The figure shows three views and two pictorial views of one solid part (mm, origin at its lowest corner). Answer the questions. Round coordinates to 2 decimals unless told otherwise and drop trailing zeros. Order: outer loops, then holes, each group sorted by start corner. A loop starts at its lowest first (then second) coordinate and runs counter-clockwise, first axis right, second up. Notation, with made-up numbers: (-23.75, 30.25) - (-5.75, 30.25) arc R31 cw to (-5.75, 60.25) - close; hole circle Ø5 at (81, 57). An arc over 180 degrees is marked (long way). Write item = value, one per line.
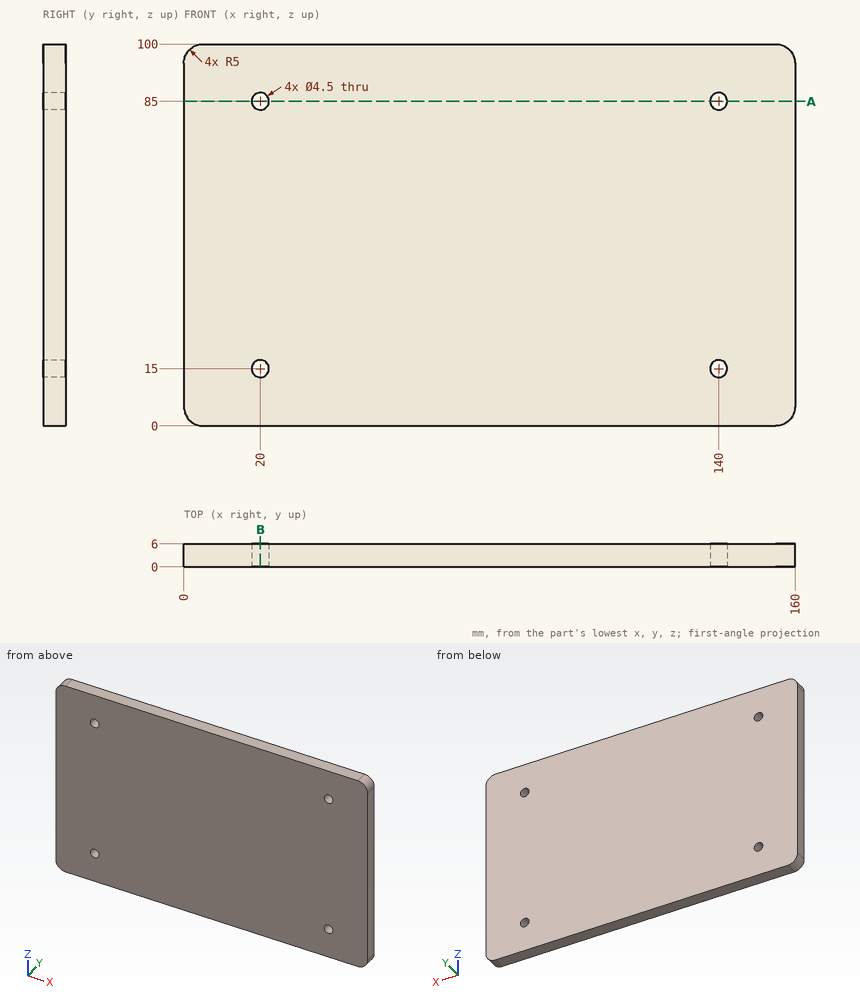
Q1. Section A-A on z = 85 is taken. Determine the outline of the cut face in (x, y).
Model answer:
outline = (0, 0) - (17.75, 0) - (17.75, 6) - (0, 6) - close; (22.25, 0) - (137.75, 0) - (137.75, 6) - (22.25, 6) - close; (142.25, 0) - (160, 0) - (160, 6) - (142.25, 6) - close
Q2. Find the intervals of material crossed by line 1 (Z direction, x = 140, y = 1.5); line 2 (X direction, y = 4, z = 15); line 3 (Z direction, x = 138.5, y = 0.5), in increasing order. Write a range as from..to.
Model answer:
line_1 = 0..12.75, 17.25..82.75, 87.25..100
line_2 = 0..17.75, 22.25..137.75, 142.25..160
line_3 = 0..13.32, 16.68..83.32, 86.68..100
Q3. Section B-B on x = 20 is taken. Determine the outline of the cut face in (y, z).
Model answer:
outline = (0, 0) - (6, 0) - (6, 12.75) - (0, 12.75) - close; (0, 17.25) - (6, 17.25) - (6, 82.75) - (0, 82.75) - close; (0, 87.25) - (6, 87.25) - (6, 100) - (0, 100) - close
Q4. A flat-ended cylindrical pin translates along its axis: P1, Ø2.5, axis at x = 140, z = 15, coming from the -Y side. Find the tip coordinate at first contact, or state that the pin passes through.
Model answer:
P1 = through
